Input: part model. Units: mm. Frame: model coordinates. Face numbers are marked on the shaded views. Round coordinates to 2 decimals unless told otherwise and drop trailing zeros. Order: outer loops, then holes, each group sorted by start corner. A loop starts at its lowest first (then second) coordinate and runs counter-clockwise, first axis right, second up. Notation, with made-up numbers: (-2.5, 48.25) -> (26.5, 48.25) arc R6 cw to (26.5, 57.25) -> close; hole circle Ø5 at (68, -3). An arc over 180 degrees is marked (long way). Use a Markdown table: item, result.
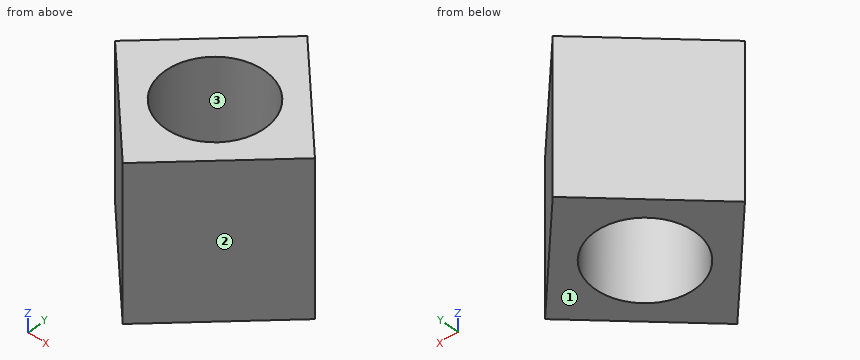
from build123d import *

# Parameters (mm, degrees)
SKETCH_1_R      = 2.1
EXTRUDE_1_DEPTH = 6.5


with BuildPart() as part:
    # ｽｹｯﾁ1 → ﾎﾞｽ - 押し出し1 (new body)
    with BuildSketch(Plane.XY):
        Polygon((4.242640687, 0), (0, 4.242640687), (-4.242640687, 0), (0, -4.242640687), align=None)
        with Locations(Location((0, 0, 0), (0, 0, 180))):
            Circle(SKETCH_1_R, mode=Mode.SUBTRACT)
    extrude(amount=EXTRUDE_1_DEPTH)


solid = part.part
1) Cut plane A-A on x = -0.25. Return loops of the section in (y, z), and give its area (3 significant figures).
Results found:
| item | result |
|---|---|
| outline | (-3.99, 0) -> (-2.09, 0) -> (-2.09, 6.5) -> (-3.99, 6.5) -> close; (2.09, 0) -> (3.99, 0) -> (3.99, 6.5) -> (2.09, 6.5) -> close |
| area | 24.8 mm² |
2) Line query: L1, parallel to X at y = -1.75, z = 3.25; L2, parallel to Y at x = 1.5, z = 5.75; L3, parallel to X at y = 0.5, z = 3.5. Output: solid intervals per line, ascending. Write a range as [from, to].
Results found:
| item | result |
|---|---|
| L1 | x = [-2.49, -1.16], [1.16, 2.49] |
| L2 | y = [-2.74, -1.47], [1.47, 2.74] |
| L3 | x = [-3.74, -2.04], [2.04, 3.74] |
3) Cut plane C-C on z = 4.5. Return loops of the section in (x, y), and give its area (3 significant figures).
Results found:
| item | result |
|---|---|
| outline | (-4.24, 0) -> (0, -4.24) -> (4.24, 0) -> (0, 4.24) -> close; hole circle Ø4.2 at (0, 0) |
| area | 22.1 mm² |
4) Pull-direction query (X, two-part tool) for the marked faces 1, 2 and 3; classes: +X half, -X half, draft (parallel to the pull), parting line (faces both ways), or undercut.
Results found:
| item | result |
|---|---|
| face 1 | draft |
| face 2 | +X half |
| face 3 | undercut |
5) Pin query (flat end, axial travel): pin 1 Ø3 at (y, z) = (-0.5, 0.5) entering from -X; pin 2 Ø2 at (y, z) = (1.5, 5) entering from -X; pin 3 Ø2 at (x, z) = (-0.5, 3.5) entering from +Y. Return the tip coordinate at first contact, or that it passes through.
Results found:
| item | result |
|---|---|
| pin 1 | stops at x = -4.24 |
| pin 2 | stops at x = -3.74 |
| pin 3 | stops at y = 4.24 |
6) Cut plane D-D on y = -3.5. Return loops of the section in (x, z), and give its area (3 significant figures).
Results found:
| item | result |
|---|---|
| outline | (-0.74, 0) -> (0.74, 0) -> (0.74, 6.5) -> (-0.74, 6.5) -> close |
| area | 9.65 mm² |
